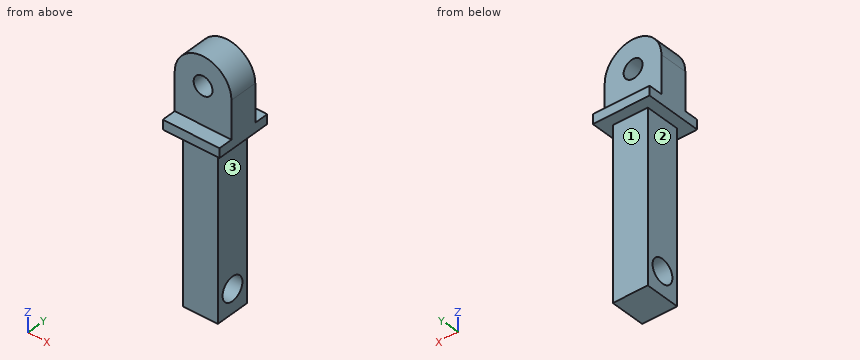
from build123d import *

# Parameters (mm, degrees)
SKETCH_1_W           = 6
SKETCH_1_H           = 6
EXTRUDE_1_DEPTH      = 1
SKETCH_2_R           = 1
EXTRUDE_2_DEPTH      = 1.5
EXTRUDE_2_DEPTH_BACK = 1.5
SKETCH_3_W           = 3.7
SKETCH_3_H           = 3.7
EXTRUDE_3_DEPTH      = 18
SKETCH_4_R           = 1.25
CUT_EXTRUDE_1_DEPTH  = 3.7


with BuildPart() as part:
    # 스케치1 → 보스-돌출1 (new body)
    with BuildSketch(Plane.XY):
        Rectangle(SKETCH_1_W, SKETCH_1_H)
    extrude(amount=EXTRUDE_1_DEPTH)

    # 스케치2 → 보스-돌출2 (add, two sides)
    with BuildSketch(Plane(origin=(0, 0, 0), x_dir=(1, 0, 0), z_dir=(0, 1, 0))) as extrude_2_sk:
        with BuildLine():
            Line((-3, -1), (3, -1))
            Line((3, -1), (3, -5))
            ThreePointArc((3, -5), (0, -8), (-3, -5))
            Line((-3, -5), (-3, -1))
        make_face()
        with Locations((0, -5)):
            Circle(SKETCH_2_R, mode=Mode.SUBTRACT)
    extrude(amount=EXTRUDE_2_DEPTH)
    extrude(extrude_2_sk.sketch, amount=-EXTRUDE_2_DEPTH_BACK)

    # 스케치3 → 보스-돌출3 (add)
    with BuildSketch(Plane(origin=(0, 0, 0), x_dir=(-1, 0, 0), z_dir=(0, 0, -1))):
        Rectangle(SKETCH_3_W, SKETCH_3_H)
    extrude(amount=EXTRUDE_3_DEPTH)

    # 스케치4 → 컷-돌출1 (cut)
    with BuildSketch(Plane.ZY.offset(1.85)):
        with Locations((-15.5, 0)):
            Circle(SKETCH_4_R)
    extrude(amount=-CUT_EXTRUDE_1_DEPTH, mode=Mode.SUBTRACT)


solid = part.part
The listing builds one solid part. Answer for the finished solid, in the listing's coordinates (mm). Face numbers are marked on the shaded views. A direction names the side the tool comes from. Give positions to 0.01 mm unless a question says otherwise; leave off trailing zeros. Write each loop counter-clockwise with the first axis right and the second up, starting at its lowest first coordinate (ties: lowest second). Pieces come first, ordered by that corner, then holes. Notation, with made-up numbers: (28, 42) -> (38, 42) arc R11 ccw to (38, 57) -> close; hole circle Ø5 at (-0.5, 26.5). An arc over 180 degrees is marked (long way). Use a Markdown table: item, result.
(1) For the marked faces 1, 2 and 3, determine the directions among +Z, -Z, +X, -X, +Y, -Y from which every point of the face is accessible in a straight line to the end or side of a thin tool.
Return value:
| item | result |
|---|---|
| face 1 | -Z, +X, -X, +Y |
| face 2 | -Z, -X, +Y, -Y |
| face 3 | -Z, +X, +Y, -Y |
(2) Section C-C, the plane y = -0.9 is taken. Determine the outline of the cut face in (x, z).
Return value:
| item | result |
|---|---|
| outline | (-3, 0) -> (-1.85, 0) -> (-1.85, -14.63) -> (1.85, -14.63) -> (1.85, 0) -> (3, 0) -> (3, 5) arc R3 ccw to (-3, 5) -> close; (-1.85, -18) -> (1.85, -18) -> (1.85, -16.37) -> (-1.85, -16.37) -> close; hole circle Ø2 at (0, 5) |
(3) Find the intervals of material crossed by probe 1 along Y at (x, z) = (-0.5, -14.75); probe 2 along Z at (x, y) = (0.2, -0.85); probe 3 along Y at (x, z) = (0.6, -15.5), in increasing order. Write a range as from..to.
Return value:
| item | result |
|---|---|
| probe 1 | -1.85..-1, 1..1.85 |
| probe 2 | -18..-16.42, -14.58..4.02, 5.98..7.99 |
| probe 3 | -1.85..-1.25, 1.25..1.85 |
(4) Section A-A, the plane x = 0 is taken. Determine the outline of the cut face in (y, z).
Return value:
| item | result |
|---|---|
| outline | (-3, 0) -> (-1.85, 0) -> (-1.85, -18) -> (1.85, -18) -> (1.85, 0) -> (3, 0) -> (3, 1) -> (1.5, 1) -> (1.5, 4) -> (-1.5, 4) -> (-1.5, 1) -> (-3, 1) -> close; (-1.5, 6) -> (1.5, 6) -> (1.5, 8) -> (-1.5, 8) -> close; hole circle Ø2.5 at (0, -15.5) |
(5) Section D-D, the plane y = -2.1 is taken. Determine the outline of the cut face in (x, z), then the cut area to 3 significant figures.
Return value:
| item | result |
|---|---|
| outline | (-3, 0) -> (3, 0) -> (3, 1) -> (-3, 1) -> close |
| area | 6.00 mm2 |
(6) Section B-B, the plane z = -15.5 is taken. Determine the outline of the cut face in (x, y), then the cut area to 3 significant figures.
Return value:
| item | result |
|---|---|
| outline | (-1.85, -1.85) -> (1.85, -1.85) -> (1.85, -1.25) -> (-1.85, -1.25) -> close; (-1.85, 1.25) -> (1.85, 1.25) -> (1.85, 1.85) -> (-1.85, 1.85) -> close |
| area | 4.44 mm2 |
(7) Flat-ended cylindrical pins translate along their axes: P1, Ø1.5, axis at x = 2, z = -1.5, coming from the +Y side; P2, Ø3, axis at y = 2, z = -5, coming from the +X side; P3, Ø2.5, axis at x = 0, z = 5, coming from the +Y side; P4, Ø2, axis at y = 0, z = -15.5, coming from the +X side. Find the tip coordinate at first contact, or state that the pin passes through.
Return value:
| item | result |
|---|---|
| P1 | y = 1.85 |
| P2 | x = 1.85 |
| P3 | y = 1.5 |
| P4 | through |
